Geometry: final body of the model. Coordinates: model frame, mm. Face numbers are marked on the shaded views. A direction names the side the tool comes from. Give positions to 0.01 mm unless a question says otherwise; leave off trailing zeros. Loops run counter-clockwise (first coordinate to the right, second up) from the corner with the lowest first, then second, coordinate; pieces in that order, holes last. Notation, with made-up numbers: (68.5, 64) - (98.5, 64) arc R19 ccw to (98.5, 92) - close; hole circle Ø5 at (28, -26.75). An arc over 180 degrees is marked (long way). Answer in a Markdown table with one row per item.
Autodesk Inventor part; units mm, degrees
ref_plane "YZ Plane" through (0, 0, 0) normal (1, 0, 0) x (0, 1, 0)
ref_plane "XZ Plane" through (0, 0, 0) normal (0, 1, 0) x (-1, 0, 0)
ref_plane "XY Plane" through (0, 0, 0) normal (0, 0, 1) x (1, 0, 0)
sketch "Sketch1" plane through (0, 0, 0) normal (0, 0, 1) x (1, 0, 0)
  circle A0 centre (0, 0) radius 2.0828
  dimension "d0" = 4.1656
extrude "Extrusion1" add sketch "Sketch1" along normal blind 9.525
sketch "Sketch2" plane through (0, 0, 0) normal (0, 1, 0) x (-1, 0, 0)
  line L0 (0, 0) -> (0, -2.2098)
  line L1 (0, 0) -> (3.9624, 0)
  line L2 (0, -2.2098) -> (2.032, -2.2098)
  line L3 (3.9624, 0) -> (3.9624, 3.6562) construction
  arc A0 (2.032, -2.2098) -> (3.9624, -0.4599) centre (0.1837, 1.7689) ccw
  line L4 (4.5847, 0.6553) -> (4.5847, -0.2608) construction
  line L5 (3.9624, -0.4599) -> (3.9624, 0)
  dimension "d3" = 2.2098
  dimension "d6" = 2.032
  dimension "d19" = 3.9624
revolve "Revolution1" add sketch "Sketch2" angle 360 about axis through (0, 0, 0) along (0, 0, -1)
sketch "Sketch3" plane through (0, 0, -2.2098) normal (0, 0, -1) x (-1, 0, 0)
  circle A0 centre (0, 0) radius 2.032
  line L0 (-0.6874, 1.1906) -> (0.6874, 1.1906)
  line L1 (0.6874, 1.1906) -> (1.3748, 0)
  line L2 (1.3748, 0) -> (0.6874, -1.1906)
  line L3 (0.6874, -1.1906) -> (-0.6874, -1.1906)
  line L4 (-0.6874, -1.1906) -> (-1.3748, 0)
  line L5 (-1.3748, 0) -> (-0.6874, 1.1906)
  dimension "d8" = 2.3813
extrude "Extrusion2" cut sketch "Sketch3" against normal blind 1.5875 contours L0 L1 L2 L3 L4 L5
chamfer "Chamfer1" distance 0.508 angle 45 1 edges at (-2.0828, 0, 9.525)
thread "Thread1"
properties part number "10-32 x500 button head" material "Steel"
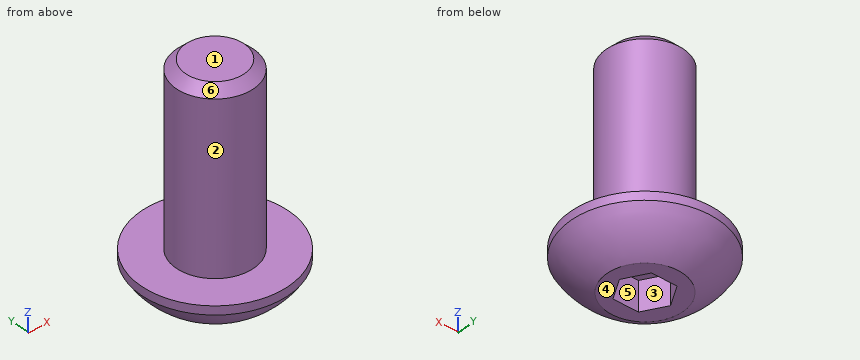
Q1. Cut plane B-B (z = -0.25). Output: boundary loops of the cut face in (x, y), and give its area (3 significant figures).
Check values:
| item | result |
|---|---|
| outline | circle Ø7.92 at (0, 0) |
| area | 49.3 mm² |
Q2. First-contact query: pin 1 (1.1 mm diameter, centred on x = 0, z = -1.5, fed in from -Y); pin 2 (1.5 mm diameter, centred on x = -1.5, z = -1, fed in from -Y); pin 3 (3 mm diameter, centred on y = -0.5, z = 2.5, fed in from -X). Flat tips, straight axial feed; report the tip coordinate or a pass-through.
Check values:
| item | result |
|---|---|
| pin 1 | y = -3.63 |
| pin 2 | y = -3.84 |
| pin 3 | x = -2.08 |
Q3. Draft query along X for the marked faces 4, 5 and 6. Return one class per face: pulls with the +X half, pulls with the -X half, needs draft (parallel to the pull), parting line crosses it, or undercut.
Check values:
| item | result |
|---|---|
| face 4 | needs draft |
| face 5 | undercut |
| face 6 | parting line crosses it |
Q4. Material intervals for line 1 along Z through (x, y) = (-1.25, -2.75); line 2 along Z through (x, y) = (0.5, 0.5) (3 decimals); line 3 along Y through (x, z) = (0.75, 4.75), sorted ascending.
Check values:
| item | result |
|---|---|
| line 1 | -1.58 to 0 |
| line 2 | -0.622 to 9.525 |
| line 3 | -1.94 to 1.94 |
Q5. Cut plane A-A (z = 4.5). Output: boundary loops of the cut face in (x, y).
Check values:
| item | result |
|---|---|
| outline | circle Ø4.17 at (0, 0) |
Q6. Reachability of the marked faces 1, 2 and 3 from +Z, -Z, +X, -X, +Y, -Y: full face, straight path, thin tool, end or side. Return the list, or none.
Check values:
| item | result |
|---|---|
| face 1 | +Z, +X, -X, +Y, -Y |
| face 2 | +Z |
| face 3 | -Z |
